Geometry: final body of the model. Coordinates: model frame, mm. A direction names the side the tool comes from. Round coordinates to 2 decimals unless told otherwise and drop trailing zeros. Loops run counter-clockwise (first coordinate to the right, second up) from the corner with the lowest first, then second, coordinate; pieces in that order, holes last. Notation, with made-up numbers: (39.25, 0.5) - (59.25, 0.5) arc R26 cw to (59.25, 35.5) - close; hole circle Ø9 at (76.5, -0.75). An arc over 180 degrees is marked (long way). Write item = value, one per line. Start each with the question number.
Item 1: Section D-D (x = 55). Return loops of the section in (y, z), plus the area to 3 significant figures.
Item 2: Line query: line 1 (Z direction, x = 80, y = 17.5); line 2 (Y direction, x = 55.5, z = 0.5); line 3 (Y direction, x = 65, z = -54). Output: solid intervals per line, ascending. Write a range as from..to.
Item 3: First-contact query: pin 1 (6 mm diameter, centred on x = 0.5, y = 0, fed in from -Z); pin 2 (1 mm diameter, centred on x = 54.5, y = 15.5, fed in from -Z); pin 3 (10 mm diameter, centred on y = -11.5, z = -19, fed in from -X); pin 4 (6.5 mm diameter, centred on x = 80, z = 5.5, fed in from -Y). Flat tips, straight axial feed; report the tip coordinate or a pass-through.
Item 4: Access query for faces 1 (the cylindrical face through (44.9, 20.01, -0.14)), 2 (the flat face through (26, 16, -20)), 3 (the cylindrical face through (47, 20, 4)). Directions: +Z, -Z, +X, -X, +Y, -Y. A direction counts if a zero-diameter tool reaches every point of the face in a straight line with its end or side. Return the directions, or none.
Item 5: Section C-C (x = 9). Return loops of the section in (y, z).
Item 6: Section A-A (x = 86). Return loops of the section in (y, z), plus the area to 3 significant figures.
Item 7: Section B-B (y = 0). Return loops of the section in (x, z).
Item 8: Draft query along Z for faces 4 (the cylindrical face through (82.4, -16.5, 3.2)), 5 (the flat face through (9, 0, -11)), 6 (the cylindrical face through (22, 0, 10)). Return one class per face: pulls with the +Z half, pulls with the -Z half, needs draft (parallel to the pull), parting line crosses it, or undercut.
from build123d import *

# Parameters (mm, degrees)
F1_DEPTH  = 16
F2_W      = 70
F2_H      = 3
F3_DEPTH  = 2
F4_W      = 50
F4_H      = 12
F5_DEPTH  = 2
F6_R      = 1
F9_DEPTH  = 2
F11_DEPTH = 42.001
F13_D     = 4
F14_R     = 3
F14_R_2   = 2
F15_DEPTH = 5
F16_R     = 3


# Not quite as in the source:
# - a pattern or mirror of a feature is missing from the dataset's text; its kind, count and spacing are read off the source's solid


with BuildPart() as f1:
    # F0 (on Front) → F1 (new body)
    with BuildSketch(Plane.XZ):
        with BuildLine():
            ThreePointArc((0, -9), (-9, 0), (0, 9))
            Line((0, 9), (94, 9))
            Line((94, 9), (94, 11))
            Line((94, 11), (0, 11))
            ThreePointArc((0, 11), (-11, 0), (0, -11))
            Line((0, -11), (19, -11))
            ThreePointArc((19, -11), (20.704090422, -11.530976745), (21.8049592536, -12.9359494441))
            ThreePointArc((21.8049592536, -12.9359494441), (42.5173607247, -42.2788136793), (74.8275397389, -57.9651003113))
            ThreePointArc((74.8275397389, -57.9651003113), (79.1628330842, -59.4937576212), (82.7692987656, -62.344190369))
            Line((82.7692987656, -62.344190369), (84.2502282886, -61))
            ThreePointArc((84.2502282886, -61), (80.1403113626, -57.7488524545), (75.200382963, -56))
            ThreePointArc((75.200382963, -56), (43.8025480023, -40.74634786), (23.6749320894, -12.2265824069))
            ThreePointArc((23.6749320894, -12.2265824069), (21.8401507033, -9.8849612416), (19, -9))
            Line((19, -9), (0, -9))
        make_face()
    extrude(amount=F1_DEPTH)

    # F2 (on face) → F3 (join)
    with BuildSketch(Plane.XY.offset(11)):
        with Locations((59, -17.5)):
            Rectangle(F2_W, F2_H)
    extrude(amount=-F3_DEPTH)

    # F4 (on face) → F5 (join)
    with BuildSketch(Plane.XZ.offset(19)):
        with Locations((69, 5)):
            Rectangle(F4_W, F4_H)
    extrude(amount=F5_DEPTH)

    # F6
    f6_edges = [f1.edges().sort_by_distance(p)[0] for p in [
        (69, -21, 11),
        (69, -19, 9),
    ]]
    fillet(f6_edges, radius=F6_R)

    # F7: F1 across plane


with BuildPart() as f1_1:
    add(f1.part)
    add(f1.part.mirror(Plane.XZ))

    # F8 (on face) → F9 (cut)
    with BuildSketch(Plane.XY.offset(11)):
        with BuildLine():
            Line((94, 12), (34, 12))
            ThreePointArc((34, 12), (22, 0), (34, -12))
            Line((34, -12), (94, -12))
            Line((94, -12), (94, 12))
        make_face()
    extrude(amount=-F9_DEPTH, mode=Mode.SUBTRACT)

    # F10 (on face) → F11 (cut, through all)
    with BuildSketch(Plane.XZ.offset(21)):
        with BuildLine():
            ThreePointArc((50, 7), (47, 4), (50, 1))
            Line((50, 1), (70, 1))
            ThreePointArc((70, 1), (73, 4), (70, 7))
            Line((70, 7), (50, 7))
        make_face()
    extrude(amount=-F11_DEPTH, mode=Mode.SUBTRACT)

    # F13 (through all)
    with Locations(Plane.XZ.offset(21)):
        with Locations((80, 5)):
            Hole(F13_D / 2)

    # F14 (on face) → F15 (join)
    with BuildSketch(Plane(origin=(0, -19, 0), x_dir=(-1, 0, 0), z_dir=(0, 1, 0))):
        with Locations((-80, 5)):
            Circle(F14_R)
        with Locations((-80, 5)):
            Circle(F14_R_2, mode=Mode.SUBTRACT)
    f15 = extrude(amount=F15_DEPTH)

    # F15_copies: F15 across plane
    add(f15.mirror(Plane.ZX))

    # F16
    f16_edges = [f1_1.edges().sort_by_distance(p)[0] for p in [
        (94, -20, -1),
        (94, 20, -1),
        (44, 20, -1),
        (44, -20, -1),
    ]]
    fillet(f16_edges, radius=F16_R)


solid = f1_1.part
Taken from the geometry:
q1.outline = (-21, -1) - (-19, -1) - (-19, 1) - (-21, 1) - close; (-21, 7) - (-19, 7) - (-19, 8) arc R1 cw to (-18, 9) - (-12, 9) - (-12, 11) - (-20, 11) arc R1 ccw to (-21, 10) - close; (-16, -50.8) - (16, -50.8) - (16, -48.52) - (-16, -48.52) - close; (12, 9) - (18, 9) arc R1 cw to (19, 8) - (19, 7) - (21, 7) - (21, 10) arc R1 ccw to (20, 11) - (12, 11) - close; (19, -1) - (21, -1) - (21, 1) - (19, 1) - close
q1.area = 125 mm^2
q2.line_1 = 2..3, 7..8, 9..11
q2.line_2 = -21..-19, 19..21
q2.line_3 = -16..16
q3.pin_1 = -11
q3.pin_2 = -50.8
q3.pin_3 = 22.22
q3.pin_4 = -21
q4.face_1 = -Z, -X, +Y, -Y
q4.face_2 = -Z, -X, +Y
q4.face_3 = +Y, -Y
q5.outline = (-16, -11) - (16, -11) - (16, -9) - (-16, -9) - close; (-16, 9) - (16, 9) - (16, 11) - (-16, 11) - close
q6.outline = (-21, -1) - (-19, -1) - (-19, 8) arc R1 cw to (-18, 9) - (-12, 9) - (-12, 11) - (-20, 11) arc R1 ccw to (-21, 10) - close; (12, 9) - (18, 9) arc R1 cw to (19, 8) - (19, -1) - (21, -1) - (21, 10) arc R1 ccw to (20, 11) - (12, 11) - close
q6.area = 76.0 mm^2
q7.outline = (0, -11) - (19, -11) arc R3 cw to (21.8, -12.94) arc R72 ccw to (74.83, -57.97) arc R14 cw to (82.77, -62.34) - (84.25, -61) arc R16 ccw to (75.2, -56) arc R70 cw to (23.67, -12.23) arc R5 ccw to (19, -9) - (0, -9) arc R9 cw to (0, 9) - (22, 9) - (22, 11) - (0, 11) arc R11 ccw to start
q8.face_4 = undercut
q8.face_5 = pulls with the -Z half
q8.face_6 = needs draft
